Geometry check sheet. Reference: the model listing, model coordinates, mm. A direction names the side the tool comes from. Give positions to 0.01 mm unless a question says otherwise; leave off trailing zeros. One line per item, written item: value. Start each with the question number.
(1) Tool access check on faces 1 (the face through (15.748, -4.959, 5.635)), 2 (the face through (0, -3, 20.32)). Record the directions out of +Z, -Z, +X, -X, +Y, -Y that give a thin tool (end or side, any length) a straight path to the whole face; none if there is none.
(2) Gauge pin test, flat ends, axial feed: pin 1 Ø5 at (x, z) = (3, 6) entering from +Y; pin 2 Ø1.5 at (x, y) = (-15.5, 4.5) entering from +Z; pin 3 Ø2 at (y, z) = (10, 3) entering from +X. Record the tip position at first contact, or that the pin passes through.
(3) Scan lines: line 1 along Y through (x, z) = (0, 12.1) (3 decimals); line 2 along Y through (x, z) = (0, 3.5); line 3 along X through (y, z) = (-4, 1.25). Record each from-to range of solid material in increasing order. Write a range as from..to.
(4) Draft check along X on faces 3 (the face through (-1.26, 0.27, 19.02)), 4 (the face through (0, 17, 0)), 5 (the face through (-2.645, -20.147, 6.261)). Enter one of: pulls with the +X half, pulls with the -X half, needs draft (parallel to the pull), parting line crosses it, or undercut.
Autodesk Inventor part; units mm, degrees
ref_plane "Work Plane1" through (0, 0, 6.35) normal (0, 0, 1) x (1, 0, 0)
ref_plane "Work Plane4" through (0, 19.1494, 6.35) normal (-1, 0, 0) x (0, -1, 0)
ref_plane "YZ Plane" through (0, 0, 0) normal (1, 0, 0) x (0, 1, 0)
sketch "Sketch1" plane through (0, 0, 0) normal (0, 0, 1) x (1, 0, 0)
  circle A0 centre (0, 0) radius 16.51
  circle A1 centre (0, 0) radius 20.32
  dimension "d0" = 40.64
  dimension "d2" = 33.02
extrude "Extrusion1" add sketch "Sketch1" along normal blind 11.43
sketch "Sketch2" plane through (0, 0, 11.43) normal (0, 0, 1) x (1, 0, 0)
  circle A0 centre (0, 0) radius 20.32
  circle A1 centre (0, 0) radius 15.875
  dimension "d5" = 31.75
extrude "Extrusion2" add sketch "Sketch2" along normal blind 1.27
fillet "Fillet1" radius 0.508 1 edges at (-15.875, 0, 11.43)
fillet "Fillet2" radius 0.508 1 edges at (-15.875, 0, 12.7)
ref_plane "Work Plane1" through (0, 0, 6.35) normal (0, 0, 1) x (1, 0, 0)
sketch "Sketch3" plane through (0, 0, 6.35) normal (0, 0, 1) x (1, 0, 0)
  line L0 (-20.32, 19.1494) -> (-20.32, -22.3588)
  circle A0 centre (0, 0) radius 20.32
  dimension "d11" = 20.32
sketch "Sketch4" plane through (0, 0, 12.7) normal (0, 0, 1) x (1, 0, 0)
  circle A0 centre (0, 0) radius 20.32
  circle A1 centre (0, 0) radius 16.383
ref_plane "Work Plane3" through (-20.32, 19.1494, 6.35) normal (-1, 0, 0) x (0, -1, 0)
ref_plane "Work Plane2" through (0, 0, 12.7) normal (0, 0, 1) x (1, 0, 0)
ref_plane "Work Plane4" through (0, 19.1494, 6.35) normal (-1, 0, 0) x (0, -1, 0)
sketch "Sketch6" plane through (0, 19.1494, 6.35) normal (-1, 0, 0) x (0, -1, 0)
  line L0 (39.364, 6.35) -> (35.554, 6.35)
  arc A0 (35.554, 6.35) -> (20.314, 11.4045) centre (19.0928, -17.78) ccw
  line L1 (39.364, 6.35) -> (39.364, 6.35)
  line L2 (31.744, 13.97) -> (20.314, 13.97)
  line L3 (20.314, 13.97) -> (20.314, 11.4045)
  arc A1 (39.364, 6.35) -> (31.744, 13.97) centre (31.744, 6.35) ccw
  line L4 (39.4694, 6.35) -> (-1.1706, 6.35)
  line L5 (19.044, 13.97) -> (19.044, 8.477)
  point P0 (19.1494, -6.35)
  point P1 (19.044, 5.9584)
  point P2 (19.044, 27.5056)
  point P3 (19.044, 11.43)
  point P4 (39.364, 13.97)
  dimension "d24" = 3.81
  dimension "d25" = 20.32
  dimension "d26" = 5.08
  dimension "d27" = 29.21
  dimension "d28" = 7.62
  dimension "d29" = 7.62
  dimension "d30" = 0
revolve "Revolution1" add sketch "Sketch6" angle 360 about axis through (0, 0.1054, 20.32) along (0, 0, -1)
properties part number "Motor End Cap" material "PVC-Piping"
Calculated:
1. face 1: -Z
1. face 2: +Z, +X, -X, +Y, -Y
2. pin 1: stops at y = 20.31
2. pin 2: stops at z = 19.84
2. pin 3: stops at x = 18.22
3. line 1: y = -20.32..-15.875, 15.875..20.32
3. line 2: y = -20.32..-16.51, 16.51..20.32
3. line 3: x = -19.92..-16.02, 16.02..19.92
4. face 3: undercut
4. face 4: needs draft
4. face 5: parting line crosses it
